from build123d import *

# Parameters (mm, degrees)
SKETCH1_R           = 2.6
SKETCH1_R_2         = 6.9
BOSS_EXTRUDE1_DEPTH = 5
BOSS_EXTRUDE2_START = 2
SKETCH2_R           = 4
SKETCH2_R_2         = 2.6
BOSS_EXTRUDE2_DEPTH = 2


with BuildPart() as part:
    # Sketch1 → Boss-Extrude1 (new body)
    with BuildSketch(Plane.XY):
        with BuildLine():
            Line((-116.116459466, -73.116163472), (-77.780395614, -32.221656848))
            ThreePointArc((-77.780395614, -32.221656848), (-76.528201342, -30.740668075), (-74.833515464, -29.797610273))
            Line((-74.833515464, -29.797610273), (-65.058269204, -23.896184603))
            ThreePointArc((-65.058269204, -23.896184603), (-61.52405595, -14.086356432), (-71.687164611, -16.417582375))
            Line((-71.687164611, -16.417582375), (-78.635941465, -22.763122171))
            ThreePointArc((-78.635941465, -22.763122171), (-81.861894444, -24.820779517), (-84.529701766, -27.563684997))
            Line((-84.529701766, -27.563684997), (-121.430579381, -63.327828505))
            ThreePointArc((-121.430579381, -63.327828505), (-132.896560675, -75.889442497), (-116.116459466, -73.116163472))
        make_face()
        with Locations((-65.969197132, -18.026447785)):
            Circle(SKETCH1_R, mode=Mode.SUBTRACT)
        with Locations((-124.987033061, -71.595333402)):
            Circle(SKETCH1_R_2, mode=Mode.SUBTRACT)
    extrude(amount=BOSS_EXTRUDE1_DEPTH)

    # Sketch2 → Boss-Extrude2 (add)
    with BuildSketch(Plane(origin=(0, 0, 0), x_dir=(-1, 0, 0), z_dir=(0, 0, -1)).offset(BOSS_EXTRUDE2_START)):
        with BuildLine():
            Line((121.430579381, -63.327828505), (84.529701766, -27.563684997))
            ThreePointArc((84.529701766, -27.563684997), (81.861894444, -24.820779517), (78.635941465, -22.763122171))
            Line((78.635941465, -22.763122171), (71.687164611, -16.417582375))
            ThreePointArc((71.687164611, -16.417582375), (61.52405595, -14.086356432), (65.058269204, -23.896184603))
            Line((65.058269204, -23.896184603), (74.833515464, -29.797610273))
            ThreePointArc((74.833515464, -29.797610273), (76.528201342, -30.740668075), (77.780395614, -32.221656848))
            Line((77.780395614, -32.221656848), (116.116459466, -73.116163472))
            ThreePointArc((116.116459466, -73.116163472), (132.896560675, -75.889442497), (121.430579381, -63.327828505))
        make_face()
        with Locations((124.987033061, -71.595333402)):
            Circle(SKETCH2_R, mode=Mode.SUBTRACT)
        with Locations((65.969197132, -18.026447785)):
            Circle(SKETCH2_R_2, mode=Mode.SUBTRACT)
    extrude(amount=-BOSS_EXTRUDE2_DEPTH)


solid = part.part
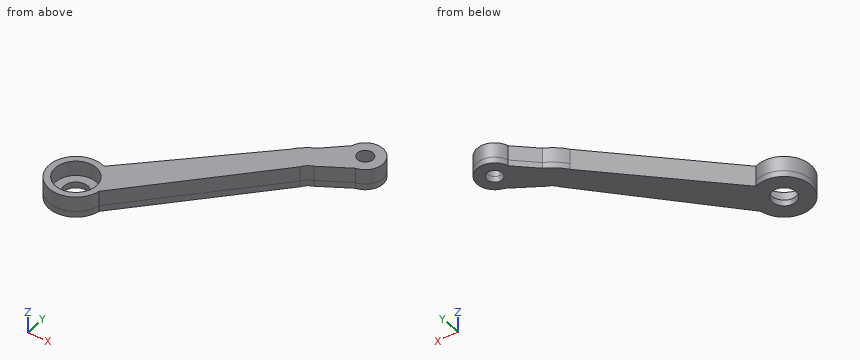
Read the model definition and answer for the solid it produces. Units are mm, in the model's axes. Round coordinates to 2 decimals unless told otherwise and drop trailing zeros. Order: outer loops, then holes, each group sorted by start corner. A loop starts at its lowest first (then second) coordinate and runs counter-clockwise, first axis right, second up.
1) Flat-ended cylindrical pins translate along their axes: pin 1 (1.5 mm diameter, centred on x = -92.5, z = 3.5, fed in from +Y); pin 2 (1 mm diameter, centred on x = -72.5, z = 1.5, fed in from -Y); pin 3 (4.5 mm diameter, centred on x = -65.97, y = -18.03, fed in from +Z); pin 4 (2 mm diameter, centred on y = -27.5, z = -0.5, fed in from +X). Find the tip coordinate at first contact, or state that the pin passes through.
2) Straight lines are drawn through the part: L1, parallel to X at y = -70, z = 2; L2, parallel to Y at x = -125, z = 3.5; L3, parallel to Y at x = -128.5, z = -0.5. For each, find the intervals that lie inside material, in ascending order.
3) The part is cut by section A-A on y = -70. Write down the section's boundary in (x, z).
4) The part is cut by section B-B on x = -125. Write down the section's boundary in (y, z).
5) The part is cut by section C-C on z = 4. Write down the section's boundary in (x, y), plus the area to 3 significant figures.
6) The part is cut by section D-D on y = -19.5. Write down the section's boundary in (x, z), plus the area to 3 significant figures.
Resolved:
1. pin 1: stops at y = -34.56
1. pin 2: stops at y = -28.69
1. pin 3: passes through
1. pin 4: stops at x = -69.37
2. L1: x = -133.84 to -131.7, -118.27 to -113.2
2. L2: y = -80.6 to -78.5, -64.7 to -62.6
2. L3: y = -79.88 to -73.51, -69.68 to -63.31
3. outline: (-133.84, -2) - (-128.66, -2) - (-128.66, 0) - (-131.7, 0) - (-131.7, 5) - (-133.84, 5) - close; (-121.32, -2) - (-113.2, -2) - (-113.2, 5) - (-118.27, 5) - (-118.27, 0) - (-121.32, 0) - close
4. outline: (-80.6, -2) - (-75.6, -2) - (-75.6, 0) - (-78.5, 0) - (-78.5, 5) - (-80.6, 5) - close; (-67.6, -2) - (-62.6, -2) - (-62.6, 5) - (-64.7, 5) - (-64.7, 0) - (-67.6, 0) - close
5. outline: (-121.43, -63.33) arc R9 ccw (long way) to (-116.12, -73.12) - (-77.78, -32.22) arc R5.4 cw to (-74.83, -29.8) - (-65.06, -23.9) arc R5.94 ccw (long way) to (-71.69, -16.42) - (-78.64, -22.76) arc R16.57 ccw to (-84.53, -27.56) - close; hole circle Ø13.8 at (-124.99, -71.6); hole circle Ø5.2 at (-65.97, -18.03)
5. area: 802 mm2
6. outline: (-75.06, -2) - (-68.11, -2) - (-68.11, 5) - (-75.06, 5) - close; (-63.83, -2) - (-60.21, -2) - (-60.21, 5) - (-63.83, 5) - close
6. area: 73.9 mm2
